from build123d import *

# Parameters (mm, degrees)
F0_R     = 40.591751
F0_W     = 49.004946
F0_H     = 18.471095
F1_DEPTH = 6.35
F2_DEPTH = 3.81


with BuildPart() as f1:
    # F0 (on Front) → F1 (new body)
    with BuildSketch(Plane.XZ):
        Circle(F0_R)
        with Locations((0, 16.86901)):
            Rectangle(F0_W, F0_H, mode=Mode.SUBTRACT)
    extrude(amount=F1_DEPTH)

    # F0 (on Front) → F2 (join)
    with BuildSketch(Plane.XZ):
        with Locations((0, 16.86901)):
            Rectangle(F0_W, F0_H)
    extrude(amount=F2_DEPTH)


solid = f1.part
CAD build for the part. Positions are in the model's coordinates, mm. A direction names the side the tool comes from. Round coordinates to 2 decimals unless told otherwise and drop trailing zeros. Order: outer loops, then holes, each group sorted by start corner. A loop starts at its lowest first (then second) coordinate and runs counter-clockwise, first axis right, second up. Notation, with made-up numbers: M 87.25,87.5 L 94.25,87.5 A36 cw 94.25,121.5 Z; hole C -13.75,53.5 d10. An arc over 180 degrees is marked long. Use one line per item in the form item = value.
Q1. Saw through at D-D on z = -8. Give the cut face in (x, y).
Recorded:
outline = M -39.8,-6.35 L 39.8,-6.35 L 39.8,0 L -39.8,0 Z
Q2. Saw through at A-A on x = 0. Give the cut face in (y, z), then the cut area to 3 significant figures.
Recorded:
outline = M -6.35,-40.59 L 0,-40.59 L 0,40.59 L -6.35,40.59 L -6.35,26.1 L -3.81,26.1 L -3.81,7.63 L -6.35,7.63 Z
area = 469 mm^2
Q3. Which spindle directions (+Z, -Z, +X, -X, +Y, -Y) get a long thin tool onto all of the face, cutting with end or side? Do faces 5 (the flat face through (0, -3.81, 17)), 6 (the flat face through (-1, -6.35, 1)). Say none if no direction does.
Recorded:
face_5 = -Y
face_6 = +Z, -Z, +X, -X, -Y
Q4. Flat gauge pins, fed straight in: P1, Ø1, axis at x = -5, y = -5, coming from the +Z side; P2, Ø3, axis at y = -5, z = 15.5, coming from the +X side; P3, Ø1.3, axis at x = 9.5, y = -5.5, coming from the +Z side. Where does each tip first touch, or does it go through?
Recorded:
P1 = 40.34
P2 = 38.1
P3 = 39.62
Q5. Saw through at C-C on x = 23. Give the cut face in (y, z), then the cut area to 3 significant figures.
Recorded:
outline = M -6.35,-33.45 L 0,-33.45 L 0,33.45 L -6.35,33.45 L -6.35,26.1 L -3.81,26.1 L -3.81,7.63 L -6.35,7.63 Z
area = 378 mm^2
Q6. Two-plate mould, pull along X, no slides. Class faces 1 (the flat face through (-1, 0, 1)), 2 (the cylindrical face through (38.72, -3.13, 12.19)), 3 (the flat face through (0, -5, 7.633)), 4 (the flat face through (-24.502, -5, 17)): +X half, -X half, draft (parallel to the pull), parting line (faces both ways), or undercut.
Recorded:
face_1 = draft
face_2 = parting line
face_3 = undercut
face_4 = undercut
Q7. Saw through at B-B on y = -2.25. Give the cut face in (x, z), then the cut area to 3 significant figures.
Recorded:
outline = C 0,0 d81.18
area = 5,180 mm^2
Q8. Probe L1, parallel to Y at x = 8, z = 21; L2, parallel to X at y = -4.5, z = 10; L3, parallel to X at y = -6, z = 21.5. List the from-to ranges inside material, lowest first.
Recorded:
L1 = -3.81 to 0
L2 = -39.34 to -24.5, 24.5 to 39.34
L3 = -34.43 to -24.5, 24.5 to 34.43
